The model under review builds one solid part; all positions refer to its coordinate system, in mm. A direction names the side the tool comes from. Round coordinates to 2 decimals unless told otherwise and drop trailing zeros. Write each loop counter-clockwise with the first axis right and the second up, starting at its lowest first coordinate (ties: lowest second). Pieces come first, ordered by that corner, then holes. Notation, with made-up numbers: (10, 42.25) - (63, 42.25) arc R26 cw to (63, 69.25) - close; hole circle Ø4 at (68, 41). An arc over 180 degrees is marked (long way). Use one line per item in the form item = value.
from build123d import *

# Parameters (mm, degrees)
SKETCH1_W           = 57.02
SKETCH1_H           = 36.2
SKETCH1_R           = 2.2
BOSS_EXTRUDE1_DEPTH = 4
SKETCH2_W           = 57.02
SKETCH2_H           = 4
BOSS_EXTRUDE2_DEPTH = 29.05
SKETCH3_W           = 4
SKETCH3_H           = 42.02
BOSS_EXTRUDE3_DEPTH = 14
SKETCH5_R           = 7
CUT_EXTRUDE1_DEPTH  = 4
SKETCH6_W           = 5
SKETCH6_H           = 18
BOSS_EXTRUDE4_DEPTH = 2.5


with BuildPart() as part:
    # Sketch1 → Boss-Extrude1 (new body)
    with BuildSketch(Plane(origin=(0, 0, 0), x_dir=(0, 0, -1), z_dir=(1, 0, 0))):
        Rectangle(SKETCH1_W, SKETCH1_H)
        with Locations((-24.51, -4.25)):
            Circle(SKETCH1_R, mode=Mode.SUBTRACT)
        with Locations((-24.51, -14.1)):
            Circle(SKETCH1_R, mode=Mode.SUBTRACT)
        with Locations((24.51, -4.25)):
            Circle(SKETCH1_R, mode=Mode.SUBTRACT)
        with Locations((24.51, -14.1)):
            Circle(SKETCH1_R, mode=Mode.SUBTRACT)
    extrude(amount=BOSS_EXTRUDE1_DEPTH)

    # Sketch2 → Boss-Extrude2 (add)
    with BuildSketch(Plane(origin=(4, 0, 0), x_dir=(0, 0, -1), z_dir=(1, 0, 0))):
        with Locations((0, 16.1)):
            Rectangle(SKETCH2_W, SKETCH2_H)
    extrude(amount=BOSS_EXTRUDE2_DEPTH)

    # Sketch3 → Boss-Extrude3 (add)
    with BuildSketch(Plane.XZ.offset(-14.1)):
        with Locations((31.05, 7.5)):
            Rectangle(SKETCH3_W, SKETCH3_H)
    extrude(amount=BOSS_EXTRUDE3_DEPTH)

    # Sketch5 → Cut-Extrude1 (cut)
    with BuildSketch(Plane(origin=(0, 18.1, 0), x_dir=(1, 0, 0), z_dir=(0, 1, 0))):
        with Locations((19, -10.79)):
            Circle(SKETCH5_R)
    extrude(amount=-CUT_EXTRUDE1_DEPTH, mode=Mode.SUBTRACT)

    # Sketch6 → Boss-Extrude4 (add)
    with BuildSketch(Plane(origin=(33.05, 0, 0), x_dir=(0, 0, -1), z_dir=(1, 0, 0))):
        with Locations((-26.01, 9.1)):
            Rectangle(SKETCH6_W, SKETCH6_H)
    extrude(amount=BOSS_EXTRUDE4_DEPTH)


solid = part.part
(1) Add section B-B on y = 15. Write out the cut boundary in (x, z), then the cut area to 3 significant figures.
Geometry results:
outline = (0, -28.51) - (33.05, -28.51) - (33.05, 23.51) - (35.55, 23.51) - (35.55, 28.51) - (0, 28.51) - close; hole circle Ø14 at (19, 10.79)
area = 1,740 mm2
(2) Add section C-C on y = -4.25. Write out the cut boundary in (x, z).
Geometry results:
outline = (0, -28.51) - (4, -28.51) - (4, -26.71) - (0, -26.71) - close; (0, -22.31) - (4, -22.31) - (4, 22.31) - (0, 22.31) - close; (0, 26.71) - (4, 26.71) - (4, 28.51) - (0, 28.51) - close
(3) The part is to be moulded in two halves that separate along X. For faces 5 (the cylindrical face through (1.972, -14.943, -26.542)), 6 (the flat face through (35.55, 9, 26)), 7 (the flat face through (18, 14.1, 0)), say which applies: +X half, -X half, draft (parallel to the pull), parting line (faces both ways), or undercut.
Geometry results:
face_5 = draft
face_6 = +X half
face_7 = undercut
(4) To check wall thickness, follow L1, parallel to Z at x = 2, y = -14; L2, parallel to Y at x = 2, z = -24; L3, parallel to X at y = 4.5, z = 14. State the ranges of each line that lie inside material, in increasing order.
Geometry results:
L1 = -28.51 to -26.71, -22.31 to 22.31, 26.71 to 28.51
L2 = -18.1 to -16.24, -11.96 to -6.39, -2.11 to 18.1
L3 = 0 to 4, 29.05 to 33.05
(5) Add section A-A on z = 24.51. Write out the cut boundary in (x, y).
Geometry results:
outline = (0, -18.1) - (4, -18.1) - (4, -16.3) - (0, -16.3) - close; (0, -11.9) - (4, -11.9) - (4, -6.45) - (0, -6.45) - close; (0, -2.05) - (4, -2.05) - (4, 14.1) - (29.05, 14.1) - (29.05, 0.1) - (35.55, 0.1) - (35.55, 18.1) - (0, 18.1) - close
(6) Insertion check: P1, Ø3, axis at x = 32.5, z = 2, coming from the -Y side; P2, Ø5, axis at x = 26.5, z = 0, coming from the -Y side; P3, Ø5, axis at y = -4.25, z = 24.51, coming from the -X side; P4, Ø3.5, axis at y = -14.1, z = 24.51, coming from the -X side. Each pin has a flat end and moves straight along its axis. Give the tip position at first contact, or say it passes through.
Geometry results:
P1 = 0.1
P2 = 14.1
P3 = 0
P4 = through
(7) Add section D-D on z = 10.79. Write out the cut boundary in (x, y), then the cut area to 3 significant figures.
Geometry results:
outline = (0, -18.1) - (4, -18.1) - (4, 14.1) - (12, 14.1) - (12, 18.1) - (0, 18.1) - close; (26, 14.1) - (29.05, 14.1) - (29.05, 0.1) - (33.05, 0.1) - (33.05, 18.1) - (26, 18.1) - close
area = 261 mm2
(8) Machinability: for faces 1 (the flat face through (32, 0.1, 8)), 2 (the flat face through (31, 7, -13.51)), 3 (the flat face through (4, -2, 0)), 4 (the flat face through (34, 9, 23.51)), which of the approach directions +Z, -Z, +X, -X, +Y, -Y give a long, thin tool a straight path to every point of the face, cutting with its end or side? Answer none if there is none.
Geometry results:
face_1 = +Z, -Z, +X, -Y
face_2 = -Z, +X, -Y
face_3 = +Z, -Z, -Y
face_4 = -Z, +X, +Y, -Y
